The model under review builds one solid part; all positions refer to its coordinate system, in mm. Face numbers are marked on the shaded views. A direction names the side the tool comes from. Coordinates: 2 decimals unless noted, no trailing zeros. Loops run counter-clockwise (first coordinate to the right, second up) from the corner with the lowest first, then second, coordinate; pieces in that order, holes last. Notation, with made-up numbers: M -9,-34 L 23,-34 A13 cw 23,-27 Z; hole C 48.5,-39.5 d6. An arc over 180 degrees is marked long. Return JSON: item names as keys, results as strings.
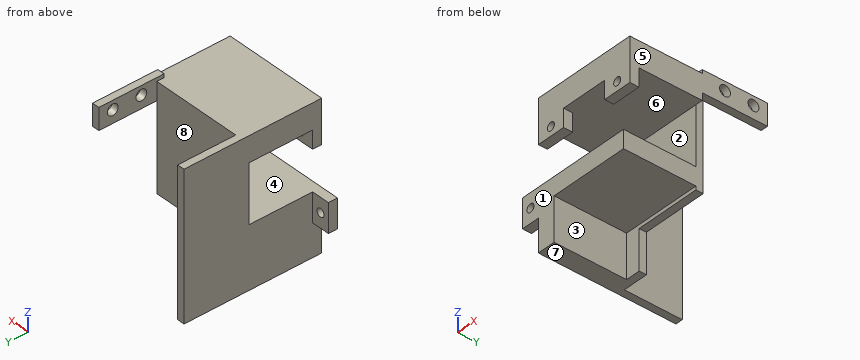
```python
from build123d import *

# Parameters (mm, degrees)
SKETCH1_W           = 31.75
SKETCH1_H           = 54.61
BOSS_EXTRUDE1_DEPTH = 2.54
SKETCH2_W           = 2.54
SKETCH2_H           = 7.62
SKETCH2_H_2         = 54.61
BOSS_EXTRUDE2_DEPTH = 22.86
SKETCH3_W           = 36.83
SKETCH3_H           = 8.89
BOSS_EXTRUDE3_DEPTH = 25.4
SKETCH4_R           = 1.905
CUT_EXTRUDE1_DEPTH  = 2.54
SKETCH5_W           = 36.83
SKETCH5_H           = 25.4
CUT_EXTRUDE2_DEPTH  = 17.78
BOSS_EXTRUDE4_DEPTH = 25.4
SKETCH7_W           = 19.05
SKETCH7_H           = 22.86
CUT_EXTRUDE3_DEPTH  = 25.4
SKETCH8_W           = 3.81
SKETCH8_H           = 48.26
CUT_EXTRUDE4_DEPTH  = 25.4
SKETCH9_W           = 10.16
SKETCH9_H           = 3.175
BOSS_EXTRUDE5_DEPTH = 6.35
SKETCH10_W          = 10.16
SKETCH10_H          = 3.175
BOSS_EXTRUDE6_DEPTH = 6.35
SKETCH11_R          = 1.4224
CUT_EXTRUDE5_DEPTH  = 77.086144107


with BuildPart() as part:
    # Sketch1 → Boss-Extrude1 (new body)
    with BuildSketch(Plane(origin=(0, 0, 0), x_dir=(1, 0, 0), z_dir=(0, 1, 0))):
        with Locations((15.875, 27.305)):
            Rectangle(SKETCH1_W, SKETCH1_H)
    extrude(amount=BOSS_EXTRUDE1_DEPTH)

    # Sketch2 → Boss-Extrude2 (add)
    with BuildSketch(Plane(origin=(0, 0, 0), x_dir=(1, 0, 0), z_dir=(0, 1, 0))):
        with Locations((33.02, 2.54)):
            Rectangle(SKETCH2_W, SKETCH2_H)
        with Locations((33.02, 52.07)):
            Rectangle(SKETCH2_W, SKETCH2_H)
        with Locations((-1.27, 27.305)):
            Rectangle(SKETCH2_W, SKETCH2_H_2)
    extrude(amount=BOSS_EXTRUDE2_DEPTH)

    # Sketch3 → Boss-Extrude3 (add)
    with BuildSketch(Plane.XZ):
        with Locations((15.875, -4.445)):
            Rectangle(SKETCH3_W, SKETCH3_H)
        with Locations((15.875, -50.165)):
            Rectangle(SKETCH3_W, SKETCH3_H)
    extrude(amount=BOSS_EXTRUDE3_DEPTH)

    # Sketch4 → Cut-Extrude1 (cut)
    with BuildSketch(Plane(origin=(34.29, 0, 0), x_dir=(0, 0, -1), z_dir=(1, 0, 0))):
        with Locations((1.85, 17.967840319)):
            Circle(SKETCH4_R)
        with Locations((1.85, 7.967840319)):
            Circle(SKETCH4_R)
        with Locations((52.76, 17.967840319)):
            Circle(SKETCH4_R)
        with Locations((52.76, 7.967840319)):
            Circle(SKETCH4_R)
    extrude(amount=-CUT_EXTRUDE1_DEPTH, mode=Mode.SUBTRACT)

    # Sketch5 → Cut-Extrude2 (cut)
    with BuildSketch(Plane(origin=(0, 0, -54.61), x_dir=(-1, 0, 0), z_dir=(0, 0, -1))):
        with Locations((-15.875, -12.7)):
            Rectangle(SKETCH5_W, SKETCH5_H)
    extrude(amount=-CUT_EXTRUDE2_DEPTH, mode=Mode.SUBTRACT)

    # Sketch6 → Boss-Extrude4 (add)
    with BuildSketch(Plane.XZ):
        Polygon((-2.54, -54.61), (3.81, -54.61), (3.81, -35.56), (31.75, -35.56), (31.75, -29.21), (1.40371894, -29.21), (-2.54, -29.21), align=None)
    extrude(amount=BOSS_EXTRUDE4_DEPTH)

    # Sketch7 → Cut-Extrude3 (cut)
    with BuildSketch(Plane(origin=(34.29, 0, 0), x_dir=(0, 0, -1), z_dir=(1, 0, 0))):
        with Locations((46.355, 11.43)):
            Rectangle(SKETCH7_W, SKETCH7_H)
    extrude(amount=-CUT_EXTRUDE3_DEPTH, mode=Mode.SUBTRACT)

    # Sketch8 → Cut-Extrude4 (cut)
    with BuildSketch(Plane.ZY.offset(2.54)):
        with Locations((-52.705, -1.27)):
            Rectangle(SKETCH8_W, SKETCH8_H)
    extrude(amount=-CUT_EXTRUDE4_DEPTH, mode=Mode.SUBTRACT)

    # Sketch9 → Boss-Extrude5 (add)
    with BuildSketch(Plane(origin=(0, 0, -8.89), x_dir=(-1, 0, 0), z_dir=(0, 0, -1))):
        with Locations((-29.21, -23.8125)):
            Rectangle(SKETCH9_W, SKETCH9_H)
        with Locations((-2.54, -23.8125)):
            Rectangle(SKETCH9_W, SKETCH9_H)
    extrude(amount=BOSS_EXTRUDE5_DEPTH)

    # Sketch10 → Boss-Extrude6 (add)
    with BuildSketch(Plane.ZY.offset(2.54)):
        with Locations((-34.29, -23.8125)):
            Rectangle(SKETCH10_W, SKETCH10_H)
    extrude(amount=BOSS_EXTRUDE6_DEPTH)

    # Sketch11 → Cut-Extrude5 (cut, through all)
    with BuildSketch(Plane(origin=(0, -22.225, 0), x_dir=(1, 0, 0), z_dir=(0, 1, 0))):
        with Locations(Location((29.21, 12.065, 0), (0, 0, 270))):
            Circle(SKETCH11_R)
        with Locations(Location((2.54, 12.065, 0), (0, 0, 270))):
            Circle(SKETCH11_R)
        with Locations(Location((-5.715, 34.29, 0), (0, 0, 270))):
            Circle(SKETCH11_R)
    extrude(amount=-CUT_EXTRUDE5_DEPTH, mode=Mode.SUBTRACT)


solid = part.part
```
1. The part is to be moulded in two halves that separate along Z. For the marked faces 6, 7 and 8, say which applies: released by +Z, released by -Z, zero draft, split by the parting line, or undercut.
Check values:
{"face 6": "undercut", "face 7": "released by -Z", "face 8": "zero draft"}
2. Insertion check: pin 1 Ø6 at (y, z) = (17.97, -1.85) entering from -X; pin 2 Ø5 at (y, z) = (-5.5, -44.5) entering from +X; pin 3 Ø1 at (x, z) = (-2.5, -28.5) entering from -Y; pin 4 Ø12.5 at (x, y) = (10, -18) entering from -Z. Each pin has a flat end and moves straight along its axis. Give the tip position at first contact, or say it passes through.
Check values:
{"pin 1": "x = -2.54", "pin 2": "x = 3.81", "pin 3": "y = 0", "pin 4": "z = -50.8"}
3. Add section A-A on z = -1.85. Give the boundary of the cut face in (x, y), plus the area to 3 significant figures.
Check values:
{"outline": "M -2.54,-25.4 L 34.29,-25.4 L 34.29,6.06 L 31.75,6.06 L 31.75,2.54 L 0,2.54 L 0,22.86 L -2.54,22.86 Z; M 31.75,9.87 L 34.29,9.87 L 34.29,16.06 L 31.75,16.06 Z; M 31.75,19.87 L 34.29,19.87 L 34.29,22.86 L 31.75,22.86 Z", "area": "1,110 mm²"}
4. Add section C-C on x = 2.54. Give the boundary of the cut face in (y, z) (3 decimals), plus the area to 3 significant figures.
Check values:
{"outline": "M -25.4,-50.8 L 2.54,-50.8 L 2.54,0 L -25.4,0 L -25.4,-10.643 L -22.225,-10.643 L -22.225,-8.89 L 0,-8.89 L 0,-29.21 L -25.4,-29.21 Z; M -25.4,-15.24 L -22.225,-15.24 L -22.225,-13.487 L -25.4,-13.487 Z", "area": "914 mm²"}
5. Add section D-D on z = -34.29. Give the boundary of the cut face in (x, y) (3 decimals), plus the area to 3 significant figures.
Check values:
{"outline": "M -8.89,-25.4 L -7.137,-25.4 L -7.137,-22.225 L -8.89,-22.225 Z; M -4.293,-25.4 L 31.75,-25.4 L 31.75,2.54 L 0,2.54 L 0,22.86 L -2.54,22.86 L -2.54,-22.225 L -4.293,-22.225 Z", "area": "1,020 mm²"}
6. Add section B-B on y = -15.5. Give the boundary of the cut face in (x, z).
Check values:
{"outline": "M -2.54,-50.8 L 3.81,-50.8 L 3.81,-35.56 L 31.75,-35.56 L 31.75,-29.21 L -2.54,-29.21 Z; M -2.54,-8.89 L 34.29,-8.89 L 34.29,0 L -2.54,0 Z"}
7. Machinability: for the marked faces 1, 2, 3, 4 and 5, which of the approach directions +Z, -Z, +X, -X, +Y, -Y give a long, thin tool a straight path to every point of the face, cutting with its end or side? Answer none if there is none.
Check values:
{"face 1": "+Z, -Z, +X, -X, -Y", "face 2": "+X, -X", "face 3": "-Z, +X, -Y", "face 4": "+X, -X, -Y", "face 5": "+Z, -Z, +X, +Y, -Y"}
8. To check wall thickness, follow line 1 (Y direction, x = 33.25, z = -1.85); line 2 (X direction, y = -22.5, z = -14.5); line 3 (Y direction, x = 33, z = -1). State the ranges of each line that lie inside material, in increasing order.
Check values:
{"line 1": "-25.4 to 6.06, 9.87 to 16.06, 19.87 to 22.86", "line 2": "-2.54 to 7.62, 24.13 to 34.29", "line 3": "-25.4 to 6.26, 9.67 to 16.26, 19.67 to 22.86"}
